Verification items for this drawing (mm, ordinates from the low corner). A direction names the side the tool comes from. Round coordinates to 2 decimals unless told otherwise and drop trailing zeros. Write each loop counter-clockwise with the first axis right and the second up, starting at its lowest first coordinate (ties: lowest second). Pieces come first, ordered by that corner, then holes. Notation, with made-up numbers: (38.25, -0.5) -> (82.25, -0.5) arc R7 ccw to (82.25, 5.5) -> close; hole circle Ø8 at (-29.5, 3.5). An arc over 180 degrees is marked (long way). One line per item, written item: value.
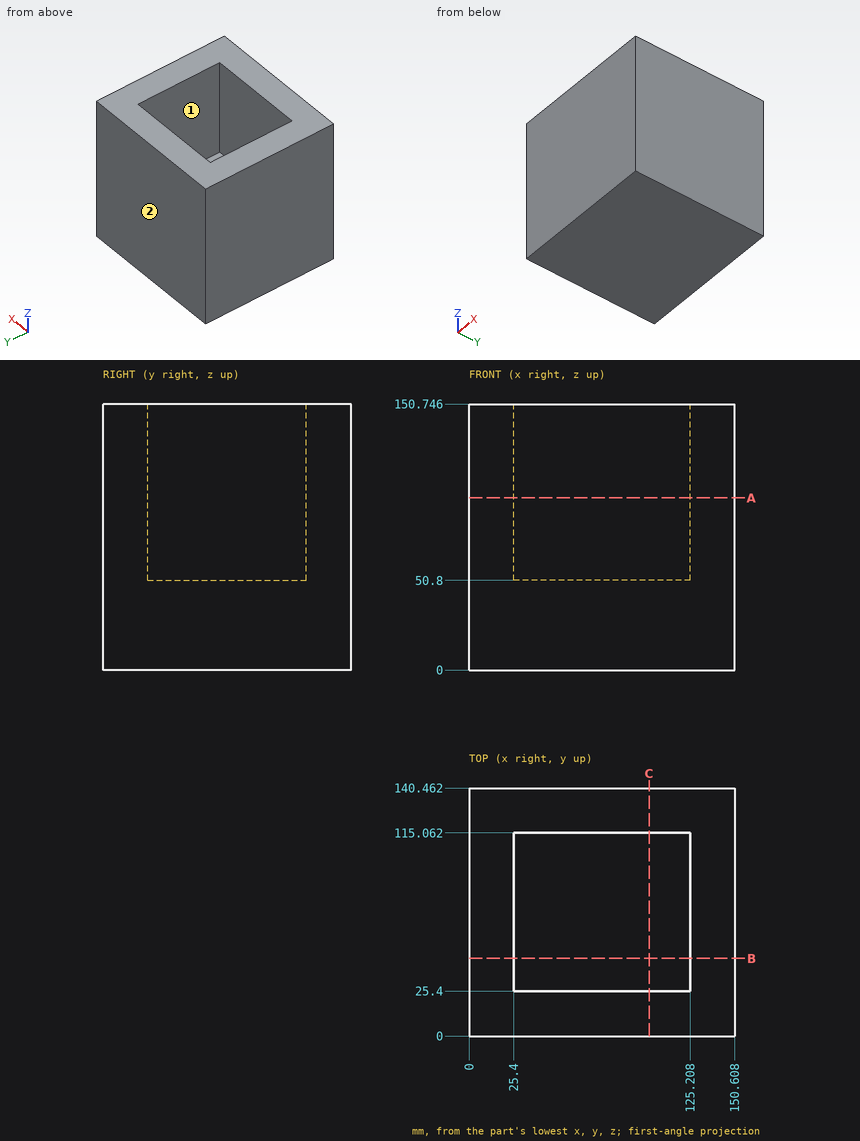
Item 1: Tool access check on the marked faces 1 and 2. Record the directions out of +Z, -Z, +X, -X, +Y, -Y that give a thin tool (end or side, any length) a straight path to the whole face; none if there is none.
Result set:
face 1: +Z
face 2: +Z, -Z, +X, -X, +Y
Item 2: Sectioned sample at B-B (y = 44). Enter the section's corners in (x, z).
Result set:
outline: (0, 0) -> (150.61, 0) -> (150.61, 150.75) -> (125.21, 150.75) -> (125.21, 50.8) -> (25.4, 50.8) -> (25.4, 150.75) -> (0, 150.75) -> close
Item 3: Depth check by flat-ended pin: pin 1 (10 mm diameter, centred on y = 64, z = 37, fed in from -X); pin 2 (4 mm diameter, centred on x = 99, y = 83, fed in from +Z). Enter the tip coordinate at first touch or a pass-through.
Result set:
pin 1: x = 0
pin 2: z = 50.8
Item 4: Sectioned sample at C-C (x = 102). Enter the section's corners in (y, z).
Result set:
outline: (0, 0) -> (140.46, 0) -> (140.46, 150.75) -> (115.06, 150.75) -> (115.06, 50.8) -> (25.4, 50.8) -> (25.4, 150.75) -> (0, 150.75) -> close
Item 5: Sectioned sample at A-A (z = 97.5). Enter the section's corners in (x, y).
Result set:
outline: (0, 0) -> (150.61, 0) -> (150.61, 140.46) -> (0, 140.46) -> close; hole (25.4, 25.4) -> (125.21, 25.4) -> (125.21, 115.06) -> (25.4, 115.06) -> close
Item 6: Material ranges on line 1 along X through (y, z) = (37.5, 77); line 2 along Y through (x, z) = (57, 96); line 3 along Z through (x, y) = (116.5, 96), recorded low to high.
Result set:
line 1: 0 to 25.4, 125.21 to 150.61
line 2: 0 to 25.4, 115.06 to 140.46
line 3: 0 to 50.8
